```python
from build123d import *

# Parameters (mm, degrees)
SKETCH1_R               = 27.125
SKETCH1_R_2             = 25.375
BOSS_EXTRUDE1_DEPTH     = 125
SKETCH5_W               = 12
SKETCH5_H               = 15
CUT_EXTRUDE1_DEPTH      = 28.125
CUT_EXTRUDE1_DEPTH_BACK = 28.125


with BuildPart() as part:
    # Sketch1 → Boss-Extrude1 (new body, symmetric)
    with BuildSketch(Plane(origin=(0, 0, 0), x_dir=(1, 0, 0), z_dir=(0, 1, 0))):
        Circle(SKETCH1_R)
        Circle(SKETCH1_R_2, mode=Mode.SUBTRACT)
    extrude(amount=BOSS_EXTRUDE1_DEPTH, both=True)

    # Sketch5 → Cut-Extrude1 (cut, two sides)
    with BuildSketch(Plane.XY) as cut_extrude1_sk:
        with Locations((0, -93.7)):
            Rectangle(SKETCH5_W, SKETCH5_H)
    extrude(amount=CUT_EXTRUDE1_DEPTH, mode=Mode.SUBTRACT)
    extrude(cut_extrude1_sk.sketch, amount=-CUT_EXTRUDE1_DEPTH_BACK, mode=Mode.SUBTRACT)


solid = part.part
```
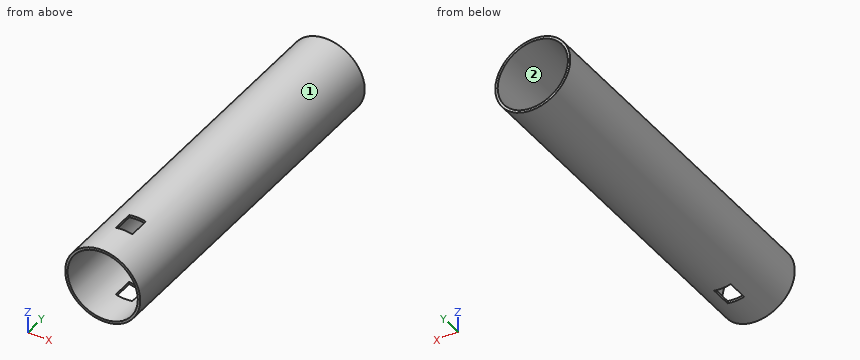
For this review, take the finished solid that the model builds, in its own axes (mm). Face numbers are marked on the shaded views. Give positions to 0.01 mm unless a question says otherwise; leave off trailing zeros. Loops run counter-clockwise (first coordinate to the right, second up) from the corner with the lowest first, then second, coordinate; pieces in that order, holes last. Notation, with made-up numbers: M -20.5,59.25 L 14.5,59.25 A5 ccw 14.5,65.25 Z; hole C -27.5,84.5 d7. An arc over 180 degrees is marked long. One line per item, written item: value. Start each with the question number.
Q1. Draft analysis for pull direction X (two halves, no side actions). For the marked faces 1 and 2, state which applies: released by +X, released by -X, zero draft, split by the parting line, or undercut.
Q2. For L1, parallel to Z at x = -6, y = -38.5; L2, parallel to Z at x = 0, y = -65 (3 decimals); L3, parallel to X at y = -97, z = -1.5, list the stretches that pass through material, from the lowest coordinate up.
Q3. Add section D-D (x = 15.5). Give the boundary of the cut face in (y, z), and give its area (3 significant figures).
Q4. Add section B-B (x = 0). Give the boundary of the cut face in (y, z) (3 decimals).
Q5. Clearance check with flat-ended pins moving along their axes: pin 1 Ø3 at (y, z) = (44.5, -18) entering from -X; pin 2 Ø1.5 at (y, z) = (-80, -14.5) entering from -X; pin 3 Ø12 at (y, z) = (99.5, 19) entering from +X. State where each tip first meets the part, or that it passes through.
Q6. Add section A-A (z = 0). Give the boundary of the cut face in (x, y) (3 decimals), and give its area (3 significant figures).
Q7. Add section C-C (y = -54). Give the boundary of the cut face in (x, z) (3 decimals), and give its area (3 significant figures).
Reply:
1. face 1: split by the parting line
1. face 2: undercut
2. L1: -26.45 to -24.66, 24.66 to 26.45
2. L2: -27.125 to -25.375, 25.375 to 27.125
2. L3: -27.08 to -25.33, 25.33 to 27.08
3. outline: M -125,-22.26 L 125,-22.26 L 125,-20.09 L -125,-20.09 Z; M -125,20.09 L 125,20.09 L 125,22.26 L -125,22.26 Z
3. area: 1,080 mm²
4. outline: M -125,-27.125 L -101.2,-27.125 L -101.2,-25.375 L -125,-25.375 Z; M -125,25.375 L -101.2,25.375 L -101.2,27.125 L -125,27.125 Z; M -86.2,-27.125 L 125,-27.125 L 125,-25.375 L -86.2,-25.375 Z; M -86.2,25.375 L 125,25.375 L 125,27.125 L -86.2,27.125 Z
5. pin 1: x = -21.53
5. pin 2: x = -23.38
5. pin 3: x = 23.81
6. outline: M -27.125,-125 L -25.375,-125 L -25.375,125 L -27.125,125 Z; M 25.375,-125 L 27.125,-125 L 27.125,125 L 25.375,125 Z
6. area: 875 mm²
7. outline: C 0,0 d54.25; hole C 0,0 d50.75
7. area: 289 mm²
